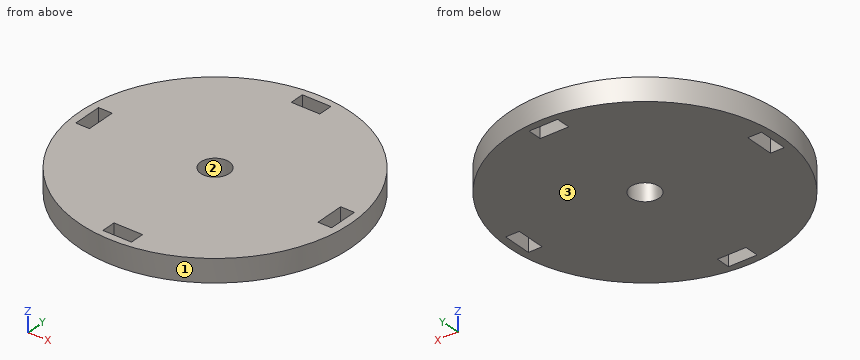
```python
from build123d import *

# Parameters (mm, degrees)
SKETCH1_R           = 11.9
BOSS_EXTRUDE1_DEPTH = 2
CUT_EXTRUDE1_REACH  = 18.948
SKETCH3_W           = 1.198540621
SKETCH3_H           = 2.563545218
CUT_EXTRUDE2_REACH  = 18.948
SKETCH4_R           = 1.25
CUT_EXTRUDE3_REACH  = 18.948
SKETCH5_W           = 2.5
SKETCH5_H           = 1.25


with BuildPart() as part:
    # Sketch1 → Boss-Extrude1 (new body)
    with BuildSketch(Plane.XY):
        Circle(SKETCH1_R)
    extrude(amount=BOSS_EXTRUDE1_DEPTH)

    # Sketch3 → Cut-Extrude1 (cut, up to next)
    with BuildSketch(Plane.XY.offset(2), mode=Mode.PRIVATE) as cut_extrude1_sk1:
        with Locations((10.59927031, 0)):
            Rectangle(SKETCH3_W, SKETCH3_H)
    cut_extrude1_tool1 = extrude(cut_extrude1_sk1.sketch, amount=-CUT_EXTRUDE1_REACH, mode=Mode.PRIVATE) & part.part
    # Sketch3 → Cut-Extrude1 (cut, up to next)
    with BuildSketch(Plane.XY.offset(2), mode=Mode.PRIVATE) as cut_extrude1_sk2:
        with Locations((-10.59927031, 0)):
            Rectangle(SKETCH3_W, SKETCH3_H)
    cut_extrude1_tool2 = extrude(cut_extrude1_sk2.sketch, amount=-CUT_EXTRUDE1_REACH, mode=Mode.PRIVATE) & part.part
    add(cut_extrude1_tool1.solids().sort_by_distance((10.59927, 0, 2))[0], mode=Mode.SUBTRACT)
    add(cut_extrude1_tool2.solids().sort_by_distance((-10.59927, 0, 2))[0], mode=Mode.SUBTRACT)

    # Sketch4 → Cut-Extrude2 (cut, up to next)
    with BuildSketch(Plane.XY.offset(2), mode=Mode.PRIVATE) as cut_extrude2_sk1:
        Circle(SKETCH4_R)
    cut_extrude2_tool1 = extrude(cut_extrude2_sk1.sketch, amount=-CUT_EXTRUDE2_REACH, mode=Mode.PRIVATE) & part.part
    add(cut_extrude2_tool1.solids().sort_by_distance((0, 0, 2))[0], mode=Mode.SUBTRACT)

    # Sketch5 → Cut-Extrude3 (cut, up to next)
    with BuildSketch(Plane(origin=(0, 0, 0), x_dir=(-1, 0, 0), z_dir=(0, 0, -1)), mode=Mode.PRIVATE) as cut_extrude3_sk1:
        with Locations((-0.161415602, -10.625)):
            Rectangle(SKETCH5_W, SKETCH5_H)
    cut_extrude3_tool1 = extrude(cut_extrude3_sk1.sketch, amount=-CUT_EXTRUDE3_REACH, mode=Mode.PRIVATE) & part.part
    # Sketch5 → Cut-Extrude3 (cut, up to next)
    with BuildSketch(Plane(origin=(0, 0, 0), x_dir=(-1, 0, 0), z_dir=(0, 0, -1)), mode=Mode.PRIVATE) as cut_extrude3_sk2:
        with Locations((-0.161415602, 10.625)):
            Rectangle(SKETCH5_W, SKETCH5_H)
    cut_extrude3_tool2 = extrude(cut_extrude3_sk2.sketch, amount=-CUT_EXTRUDE3_REACH, mode=Mode.PRIVATE) & part.part
    add(cut_extrude3_tool1.solids().sort_by_distance((0.161416, -10.625, 0))[0], mode=Mode.SUBTRACT)
    add(cut_extrude3_tool2.solids().sort_by_distance((0.161416, 10.625, 0))[0], mode=Mode.SUBTRACT)


solid = part.part
```
The model under review builds one solid part; all positions refer to its coordinate system, in mm. Face numbers are marked on the shaded views. Round coordinates to 2 decimals unless told otherwise and drop trailing zeros. Order: outer loops, then holes, each group sorted by start corner. A loop starts at its lowest first (then second) coordinate and runs counter-clockwise, first axis right, second up.
(1) Take a section at C-C, the plane x = 0.5. State the section outline as (y, z) points, plus the area to 3 significant figures.
Working result:
outline: (-11.89, 0) - (-11.25, 0) - (-11.25, 2) - (-11.89, 2) - close; (-10, 0) - (-1.15, 0) - (-1.15, 2) - (-10, 2) - close; (1.15, 0) - (10, 0) - (10, 2) - (1.15, 2) - close; (11.25, 0) - (11.89, 0) - (11.89, 2) - (11.25, 2) - close
area: 38.0 mm2
(2) Mouldability with a two-part tool opening along X and no side actions: class the marked faces 1, 2 and 3 as released by +X, released by -X, zero draft, split by the parting line, or undercut.
Working result:
face 1: split by the parting line
face 2: undercut
face 3: zero draft
(3) Take a section at A-A, the plane y = 0. State the section outline as (x, z) points.
Working result:
outline: (-11.9, 0) - (-11.2, 0) - (-11.2, 2) - (-11.9, 2) - close; (-10, 0) - (-1.25, 0) - (-1.25, 2) - (-10, 2) - close; (1.25, 0) - (10, 0) - (10, 2) - (1.25, 2) - close; (11.2, 0) - (11.9, 0) - (11.9, 2) - (11.2, 2) - close
(4) Wall thickness on L1, parallel to Y at x = 0, z = 1.55; L2, parallel to X at y = -0.75, z = 0.25; L3, parallel to Y at x = -0.75, z = 1.3: over which ranges is each line inside the solid? List them lowest first.
Working result:
L1: y = -11.9 to -11.25, -10 to -1.25, 1.25 to 10, 11.25 to 11.9
L2: x = -11.88 to -11.2, -10 to -1, 1 to 10, 11.2 to 11.88
L3: y = -11.88 to -11.25, -10 to -1, 1 to 10, 11.25 to 11.88
(5) Take a section at D-D, the plane x = -5.75. State the section outline as (y, z) points.
Working result:
outline: (-10.42, 0) - (10.42, 0) - (10.42, 2) - (-10.42, 2) - close
(6) For P1, Ø1, axis at x = 11, z = 1, coming from the -Y side; P2, Ø0.6, axis at x = -11, z = 1, coming from the -Y side, all flat-tipped, find the tip position at first contact; note any pin that passes through.
Working result:
P1: stops at y = -5.6
P2: stops at y = -5.21
(7) Take a section at B-B, the plane z = 0.9. State the section outline as (x, y) points.
Working result:
outline: circle Ø23.8 at (0, 0); hole (-11.2, -1.28) - (-10, -1.28) - (-10, 1.28) - (-11.2, 1.28) - close; hole circle Ø2.5 at (0, 0); hole (-1.09, -11.25) - (1.41, -11.25) - (1.41, -10) - (-1.09, -10) - close; hole (-1.09, 10) - (1.41, 10) - (1.41, 11.25) - (-1.09, 11.25) - close; hole (10, -1.28) - (11.2, -1.28) - (11.2, 1.28) - (10, 1.28) - close
